Part model, mm, in its own coordinate system. Give positions to 0.01 mm unless a question says otherwise; leave off trailing zeros. Write each loop counter-clockwise with the first axis right and the second up, starting at its lowest first coordinate (ties: lowest second). Pieces come first, ordered by that corner, then holes. Notation, with made-up numbers: M -17,52 L 12,52 A7 cw 12,62 Z; hole C -25,36 d8. An arc over 180 degrees is marked long. Answer as CSV lines item,"result". Start each with the question number.
Item 1: Band-saw the part on C-C, the plane z = -5. List the corners of the cut face in (x, y).
Item 2: Wall check: L1, parallel to X at y = 0.65, z = -5; L2, parallel to X at y = 0.55, z = -5.75; L3, parallel to Z at x = -23.5, y = 2.4. Give the ranges that are in metal, low to high. Write a range as from..to.
Item 3: Pin check, flat tips, straight feed: pin 1 (3 mm diameter, centred on x = -24.5, z = -5, fed in from +Y); pin 2 (4 mm diameter, centred on x = -4, z = -5, fed in from +Y). Stop position of each tip, or through.
Item 4: Band-saw the part on B-B, the plane y = 2.55. List the corners of the cut face in (x, z), then the cut area to 3 significant figures.
Item 5: Band-saw the part on A-A, the plane x = -4. List the corners of the cut face in (y, z).
Item 6: Two-plate mould, pull along X, no slides. Class faces 1 (the cylindrical face through (-14.05, 4.699, -0.285)), 2 (the cylindrical face through (-2.414, 1.726, -5.208)), 3 (the cylindrical face through (-28.215, 4.699, -5.07)): +X half, -X half, draft (parallel to the pull), parting line (faces both ways), or undercut.
from build123d import *

# Parameters (mm, degrees)
SKETCH1_W           = 28.5
SKETCH1_H           = 10
SKETCH1_R           = 1.6
BOSS_EXTRUDE1_DEPTH = 5
FILLET1_R           = 1
CHAMFER1_SIZE       = 1.5


with BuildPart() as part:
    # Sketch1 → Boss-Extrude1 (new body)
    with BuildSketch(Plane(origin=(0, 0, 0), x_dir=(1, 0, 0), z_dir=(0, 1, 0))):
        with Locations((-14.25, 5)):
            Rectangle(SKETCH1_W, SKETCH1_H)
        with Locations(Location((-4, 5, 0), (0, 0, 270))):
            Circle(SKETCH1_R, mode=Mode.SUBTRACT)
        with Locations(Location((-24.5, 5, 0), (0, 0, 270))):
            Circle(SKETCH1_R, mode=Mode.SUBTRACT)
    extrude(amount=BOSS_EXTRUDE1_DEPTH)

    # Fillet1
    fillet1_edges = [part.edges().sort_by_distance(p)[0] for p in [
        (-28.5, 5, -5),
        (-14.25, 5, 0),
        (0, 5, -5),
        (-14.25, 5, -10),
    ]]
    fillet(fillet1_edges, radius=FILLET1_R)

    # Chamfer1
    # the kernel refuses this chamfer: 1.5 mm, written as the material it takes off along each edge
    with BuildSketch(Plane(origin=(-4, 5, -5), x_dir=(0, 0, 1), z_dir=(-1, 0, 0))) as chamfer1_piece_1:
        Polygon((1.6 + CHAMFER1_SIZE, 0), (1.6, -CHAMFER1_SIZE), (1.6, 0), align=None)
    revolve(axis=Axis((-4, 5, -5), (0, 1, 0)), mode=Mode.SUBTRACT)
    with BuildSketch(Plane(origin=(-24.5, 5, -5), x_dir=(0, 0, 1), z_dir=(-1, 0, 0))) as chamfer1_piece_2:
        Polygon((1.6 + CHAMFER1_SIZE, 0), (1.6, -CHAMFER1_SIZE), (1.6, 0), align=None)
    revolve(axis=Axis((-24.5, 5, -5), (0, 1, 0)), mode=Mode.SUBTRACT)


solid = part.part
Output:
1,outline,"M -28.5,0 L -26.1,0 L -26.1,3.5 L -27.6,5 A1 ccw -28.5,4 Z; M -22.9,0 L -5.6,0 L -5.6,3.5 L -7.1,5 L -21.4,5 L -22.9,3.5 Z; M -2.4,0 L 0,0 L 0,4 A1 ccw -0.9,5 L -2.4,3.5 Z"
2,L1,"-28.5..-26.1, -22.9..-5.6, -2.4..0"
2,L2,"-28.5..-25.91, -23.09..-5.41, -2.59..0"
2,L3,"-10..-6.25, -3.75..0"
3,pin 1,"through"
3,pin 2,"y = 3.9"
4,outline,"M -28.5,-10 L 0,-10 L 0,0 L -28.5,0 Z; hole C -24.5,-5 d3.2; hole C -4,-5 d3.2"
4,area,"269 mm²"
5,outline,"M 0,-10 L 4,-10 A1 ccw 5,-9 L 5,-8.1 L 3.5,-6.6 L 0,-6.6 Z; M 0,-3.4 L 3.5,-3.4 L 5,-1.9 L 5,-1 A1 ccw 4,0 L 0,0 Z"
6,face 1,"draft"
6,face 2,"undercut"
6,face 3,"-X half"
